Autodesk Inventor part; units mm, degrees
ref_plane "YZ Plane" through (0, 0, 0) normal (1, 0, 0) x (0, 1, 0)
ref_plane "XZ Plane" through (0, 0, 0) normal (0, 1, 0) x (-1, 0, 0)
ref_plane "XY Plane" through (0, 0, 0) normal (0, 0, 1) x (1, 0, 0)
sketch "Skizze1" plane through (0, 0, 0) normal (1, 0, 0) x (0, 1, 0)
  line L0 (0, 0) -> (0, -25)
  line L1 (0, 0) -> (16, 0)
  line L2 (16, 0) -> (16, -39)
  line L3 (9, -46) -> (-7, -46)
  arc A0 (-7, -32) -> (0, -25) centre (-7, -25) ccw
  line L4 (-7, -46) -> (-7, -32)
  arc A1 (9, -46) -> (16, -39) centre (9, -39) ccw
  circle A2 centre (0, -39) radius 7 construction
  circle A3 centre (0, -39) radius 1.7
  arc A4 (9, -11) -> (7, -13) centre (9, -13) ccw
  line L5 (9, -11) -> (16, -11)
  line L6 (7, -13) -> (7, -46)
  arc A5 (-7, -39) -> (7, -39) centre (0, -39) ccw
  arc A6 (15, -11) -> (16, -10) centre (15, -10) ccw
  dimension "d2" = 14
  dimension "d3" = 16
  dimension "d7" = 14
  dimension "d8" = 3.4
  dimension "d11" = 39
  dimension "d15" = 11
  dimension "d16" = 2
  dimension "d24" = 1
extrude "Extrusion1" add sketch "Skizze1" along normal mid plane 38 contours L1 L2 A6 L5 A4 L6 A5 L4 A0 L0
sketch "Skizze2" plane through (19, 16, -11) normal (0, 0, -1) x (-1, 0, 0)
  line L0 (0, -7) -> (0, -1)
  line L1 (38, -7) -> (0, -7)
  line L2 (38, -1) -> (38, -7)
  line L3 (19, -1) -> (19, -7) construction
  line L4 (38, -7) -> (0, -7)
  circle A0 centre (6.5, -4) radius 1.7
  circle A1 centre (31.5, -4) radius 1.7
  circle A2 centre (6.5, -4) radius 3
  circle A3 centre (31.5, -4) radius 3
  line L5 (38, -1) -> (0, -1)
  point P0 (19, -16)
  dimension "d17" = 3.4
  dimension "d18" = 6
  dimension "d19" = 25
extrude "Extrusion2" cut sketch "Skizze2" against normal through all contours A0 | A1
extrude "Extrusion3" cut sketch "Skizze2" against normal blind 4 contours A2 | A3
equation "\"d2\" = d7"
properties part number "Skirt Mount" material "ABS-Kunststoff"
Model file for the job. Use its own axes, mm. A direction names the side the tool comes from. Coordinates: 2 decimals unless noted, no trailing zeros. Order: outer loops, then holes, each group sorted by start corner. A loop starts at its lowest first (then second) coordinate and runs counter-clockwise, first axis right, second up. Notation, with made-up numbers: (30, 12) -> (49, 12) arc R13 cw to (49, 24) -> close; hole circle Ø6 at (37.25, 21.5). An arc over 180 degrees is marked (long way). Answer as a JSON object with one key per item and string values. Group by question number.
1) Which spindle directions (+Z, -Z, +X, -X, +Y, -Y) get a long thin tool onto all of the face, cutting with end or side? Do faces 5 (the face through (-10.1, 10.2, -9)), 6 (the face through (0, 0, -12)), 7 (the face through (0, 0, -46)), 8 (the face through (0, 12, -11)). Say none if no direction does.
2) Drill centre lines: L1, parallel to X at y = 12, z = -10.1; L2, parallel to Y at x = 12.5, z = -1.25; L3, parallel to Y at x = -12.5, z = -8.4. Where is each one in solid material? Low to high.
3) Cut at A-A, the plane y = 12. Write the cut outline in (x, z), then the cut area to 3 significant figures.
4) Cut at D-D, the plane y = -3.5. Write the cut outline in (x, z).
5) Pull direction X, two halves, no side cores. Call faces 1 (the face through (10.5, 12, -7)), 2 (the face through (-19, 4, -23)), 3 (the face through (0, -7, -36)), 4 (the face through (19, 4, -23)): +X half, -X half, draft (parallel to the pull), parting line (faces both ways), or undercut.
6) Flat gauge pins, fed straight in: pin 1 (8 mm diameter, centred on x = 0.5, z = -22.5, fed in from -Y); pin 2 (8 mm diameter, centred on x = -12.5, y = 12, fed in from -Z); pin 3 (1 mm diameter, centred on x = -1, z = -36.5, fed in from +Y). Where does each tip first touch, or does it go through?
7) Cut at B-B, the plane x = -6.5. Write the cut outline in (y, z), then the cut area to 3 significant figures.
8) Cut at C-C, the plane z = -29. Write the cut outline in (x, y), then the cut area to 3 significant figures.
Check values:
{
 "1": {"face 5": "-Z", "face 6": "+Z, +X, -X, -Y", "face 7": "-Z, +X, -X", "face 8": "-Z, +X, -X, +Y"},
 "2": {"L1": "x = -19 to -15.5, -9.5 to 9.5, 15.5 to 19", "L2": "y = 0 to 10.3, 13.7 to 16", "L3": "y = 0 to 9, 15 to 16"},
 "3": {"outline": "(-19, -11) -> (-15.5, -11) -> (-15.5, -7) -> (-14.2, -7) -> (-14.2, 0) -> (-19, 0) -> close; (-10.8, -7) -> (-9.5, -7) -> (-9.5, -11) -> (9.5, -11) -> (9.5, -7) -> (10.8, -7) -> (10.8, 0) -> (-10.8, 0) -> close; (14.2, -7) -> (15.5, -7) -> (15.5, -11) -> (19, -11) -> (19, 0) -> (14.2, 0) -> close", "area": "322 mm²"},
 "4": {"outline": "(-19, -45.06) -> (19, -45.06) -> (19, -31.06) -> (-19, -31.06) -> close"},
 "5": {"face 1": "undercut", "face 2": "-X half", "face 3": "draft", "face 4": "+X half"},
 "6": {"pin 1": "stops at y = -0.16", "pin 2": "stops at z = -11.27", "pin 3": "stops at y = 7"},
 "7": {"outline": "(-7, -39) arc R7 ccw to (7, -39) -> (7, -13) arc R2 cw to (9, -11) -> (15, -11) arc R1 ccw to (16, -10) -> (16, 0) -> (0, 0) -> (0, -25) arc R7 cw to (-7, -32) -> close; hole circle Ø3.4 at (0, -39)", "area": "500 mm²"},
 "8": {"outline": "(-19, -1.26) -> (19, -1.26) -> (19, 7) -> (-19, 7) -> close", "area": "314 mm²"}
}
